For this review, take the finished solid that the model builds, in its own axes (mm). A direction names the side the tool comes from. Coordinates: 2 decimals unless noted, no trailing zeros. Order: outer loops, then holes, each group sorted by start corner. A loop starts at its lowest first (then second) coordinate and runs counter-clockwise, first axis right, second up. Notation, with made-up numbers: (33.25, -22.75) -> (69.25, -22.75) arc R14 cw to (69.25, -16.75) -> close; hole circle Ø11 at (38, 58.25). An arc over 180 degrees is marked (long way). Write item = value, one per line. Start each with the question number.
1) Insertion check: pin 1 Ø10 at (y, z) = (9.5, -6) entering from +X; pin 2 Ø2 at (x, z) = (1.5, -11.5) entering from +Y; pin 3 Ø7 at (x, z) = (4, 2.5) entering from +Y. Each pin has a flat end and moves straight along its axis. Give the tip position at first contact, or say it passes through.
2) Consider section B-B on x = -7.5. Give the boundary of the cut face in (y, z), and give its area (3 significant figures).
3) Wall thickness on probe 1 along X at (y, z) = (1.05, -3.25); probe 2 along X at (y, z) = (0.9, -10.75); probe 3 along Z at (x, y) = (-10, 1.6): over which ranges is each line inside the solid? List them lowest first. Write a range as [from, to].
4) Consider section A-A on z = -3.25. Give the boundary of the cut face in (x, y), and give its area (3 significant figures).
5) Draft analysis for pull direction Z (two halves, no side actions). For faces 4 (the face through (-5.79, 0.77, -2.87)), 5 (the face through (6, 12.06, -11)), 6 (the face through (0, -1, 7.25)), state which applies: +Z half, -Z half, draft (parallel to the pull), parting line (faces both ways), or undercut.
6) Consider section D-D on z = -10.75. Give the boundary of the cut face in (x, y).
7) Consider section C-C on y = 9.25. Give the boundary of the cut face in (x, z).
8) Machinability: for faces 1 (the face through (-11, 4.06, -9)), 2 (the face through (0, 1.56, 0)), 3 (the face through (-8, 0, -6)), which of the approach directions +Z, -Z, +X, -X, +Y, -Y give a long, thin tool a straight path to every point of the face, cutting with its end or side? Answer none if there is none.
from build123d import *

# Parameters (mm, degrees)
SKETCH1_R           = 1.75
BOSS_EXTRUDE1_DEPTH = 1.56
SKETCH2_R           = 1.75
BOSS_EXTRUDE2_DEPTH = 2.5
SKETCH3_W           = 14
SKETCH3_H           = 7
BOSS_EXTRUDE3_DEPTH = 8
SKETCH4_W           = 8.26
SKETCH4_H           = 7
CUT_EXTRUDE1_DEPTH  = 8
BOSS_EXTRUDE4_DEPTH = 5


with BuildPart() as part:
    # Sketch1 → Boss-Extrude1 (new body)
    with BuildSketch(Plane(origin=(0, 0, 0), x_dir=(1, 0, 0), z_dir=(0, 1, 0))):
        with BuildLine():
            Line((-10, 14.25), (10, 14.25))
            ThreePointArc((10, 14.25), (13.5, 10.75), (10, 7.25))
            Line((10, 7.25), (10, -7.25))
            Line((10, -7.25), (-10, -7.25))
            Line((-10, -7.25), (-10, 7.25))
            ThreePointArc((-10, 7.25), (-13.5, 10.75), (-10, 14.25))
        make_face()
        with Locations(Location((-10, 10.75, 0), (0, 0, 90))):
            Circle(SKETCH1_R, mode=Mode.SUBTRACT)
        with Locations(Location((10, 10.75, 0), (0, 0, 90))):
            Circle(SKETCH1_R, mode=Mode.SUBTRACT)
        with Locations(Location((-7.5, 3.25, 0), (0, 0, 90))):
            Circle(SKETCH1_R, mode=Mode.SUBTRACT)
        with Locations(Location((7.5, 3.25, 0), (0, 0, 90))):
            Circle(SKETCH1_R, mode=Mode.SUBTRACT)
    extrude(amount=BOSS_EXTRUDE1_DEPTH)

    # Sketch2 → Boss-Extrude2 (add)
    with BuildSketch(Plane(origin=(0, 1.56, 0), x_dir=(1, 0, 0), z_dir=(0, 1, 0))):
        with BuildLine():
            Line((-10, 14.25), (10, 14.25))
            ThreePointArc((10, 14.25), (13.5, 10.75), (10, 7.25))
            Line((10, 7.25), (-10, 7.25))
            ThreePointArc((-10, 7.25), (-13.5, 10.75), (-10, 14.25))
        make_face()
        with Locations(Location((-10, 10.75, 0), (0, 0, 90))):
            Circle(SKETCH2_R, mode=Mode.SUBTRACT)
        with Locations(Location((10, 10.75, 0), (0, 0, 90))):
            Circle(SKETCH2_R, mode=Mode.SUBTRACT)
    extrude(amount=BOSS_EXTRUDE2_DEPTH)

    # Sketch3 → Boss-Extrude3 (add)
    with BuildSketch(Plane(origin=(0, 4.06, 0), x_dir=(1, 0, 0), z_dir=(0, 1, 0))):
        with Locations((0, 10.75)):
            Rectangle(SKETCH3_W, SKETCH3_H)
    extrude(amount=BOSS_EXTRUDE3_DEPTH)

    # Sketch4 → Cut-Extrude1 (cut)
    with BuildSketch(Plane(origin=(0, 12.06, 0), x_dir=(1, 0, 0), z_dir=(0, 1, 0))):
        with Locations((0, 10.75)):
            Rectangle(SKETCH4_W, SKETCH4_H)
    extrude(amount=-CUT_EXTRUDE1_DEPTH, mode=Mode.SUBTRACT)

    # Sketch5 → Boss-Extrude4 (add)
    with BuildSketch(Plane.XZ):
        Polygon((-5.285984698, -7.25), (-5.285984698, -14.25), (5.285984698, -14.25), (5.285984698, -7.25), (5.285984698, 7.25), (-5.285984698, 7.25), align=None)
    extrude(amount=BOSS_EXTRUDE4_DEPTH)


solid = part.part
Answer sheet:
q1.pin_1 = 7
q1.pin_2 = 4.06
q1.pin_3 = 1.56
q2.outline = (0, -14.25) -> (4.06, -14.25) -> (4.06, -7.25) -> (1.56, -7.25) -> (1.56, -5) -> (0, -5) -> close; (0, -1.5) -> (1.56, -1.5) -> (1.56, 7.25) -> (0, 7.25) -> close
q2.area = 45.6 mm2
q3.probe_1 = [-10, -9.25], [-5.75, 5.75], [9.25, 10]
q3.probe_2 = [-13.5, -11.75], [-8.25, 8.25], [11.75, 13.5]
q3.probe_3 = [-14.25, -12.5], [-9, -7.25]
q4.outline = (-10, 0) -> (-9.25, 0) -> (-9.25, 1.56) -> (-10, 1.56) -> close; (-5.75, 0) -> (-5.29, 0) -> (-5.29, -5) -> (5.29, -5) -> (5.29, 0) -> (5.75, 0) -> (5.75, 1.56) -> (-5.75, 1.56) -> close; (9.25, 0) -> (10, 0) -> (10, 1.56) -> (9.25, 1.56) -> close
q4.area = 73.1 mm2
q5.face_4 = undercut
q5.face_5 = draft
q5.face_6 = +Z half
q6.outline = (-13.5, 0) -> (-11.75, 0) -> (-11.75, 4.06) -> (-13.5, 4.06) -> close; (-8.25, 0) -> (-5.29, 0) -> (-5.29, -5) -> (5.29, -5) -> (5.29, 0) -> (8.25, 0) -> (8.25, 4.06) -> (7, 4.06) -> (7, 12.06) -> (4.13, 12.06) -> (4.13, 4.06) -> (-4.13, 4.06) -> (-4.13, 12.06) -> (-7, 12.06) -> (-7, 4.06) -> (-8.25, 4.06) -> close; (11.75, 0) -> (13.5, 0) -> (13.5, 4.06) -> (11.75, 4.06) -> close
q7.outline = (-7, -14.25) -> (-4.13, -14.25) -> (-4.13, -7.25) -> (-7, -7.25) -> close; (4.13, -14.25) -> (7, -14.25) -> (7, -7.25) -> (4.13, -7.25) -> close
q8.face_1 = +Z, -Z, -X, +Y
q8.face_2 = +Z, +X, -X, +Y
q8.face_3 = +Z, -Z, -X, -Y
